For this review, take the finished solid that the model builds, in its own axes (mm). A direction names the side the tool comes from. Coordinates: 2 decimals unless noted, no trailing zeros. Loops run counter-clockwise (first coordinate to the right, second up) from the corner with the lowest first, then second, coordinate; pieces in that order, holes last.
1. Machinability: for faces 1 (the face through (-28.314, -11.099, -1.075)), 2 (the face through (37.676, 0.154, -22.737)), 3 (the face through (1, -1, -22)), which of the approach directions +Z, -Z, +X, -X, +Y, -Y give a long, thin tool a straight path to every point of the face, cutting with its end or side? Answer none if there is none.
2. Mouldability with a two-part tool opening along Z and no side actions: class faces 4 (the face through (23.38, 5.96, 8.44)), 5 (the face through (-31.66, 0.15, -22.96)), 6 (the face through (-0.27, -1.22, 18.77)) as pulls with the +Z half, pulls with the -Z half, needs draft (parallel to the pull), parting line crosses it, or undercut.
3. Take a section at B-B, the plane y = 0. Count the separate pieces of the cut face and the enclosed holes in it, then the cut area to 3 significant figures.
4. Clearance check with flat-ended pins moving along their axes: P1, Ø1.5, axis at y = 11, z = -7, coming from the -X side; P2, Ø6, axis at y = 4.5, z = 18.5, coming from the +X side; P3, Ø5.5, axis at x = 0, y = 0, coming from the -Z side. State where each tip first meets the part, or that it passes through.
5. To check wall thickness, follow probe 1 along Z at (x, y) = (0, 6); probe 2 along Z at (x, y) = (0, 1.75); probe 3 along X at (y, z) = (-12.7, 0). State the ranges of each line that lie inside material, in increasing order.
6. Take a section at A-A, the plane x = 0. State the section outline as (y, z) points.
```python
from build123d import *

# Parameters (mm, degrees)
SKETCH1_R               = 15.5
BOSS_EXTRUDE1_DEPTH     = 14
MOVE_START              = -14
MOVE_FACE1_DEPTH        = 28
CUT_EXTRUDE2_REACH      = 60.181
CUT_EXTRUDE2_END_RADIUS = 8.25
SKETCH5_R               = 2
SKETCH7_R               = 1.25
CUT_EXTRUDE3_DEPTH      = 68.268120394
FILLET1_R               = 8
CHAMFER1_SIZE           = 3
SKETCH8_R               = 3
CUT_EXTRUDE4_DEPTH      = 2


# Read off the part's stored shape, not the designer's step: Move Face1
with BuildPart() as part:
    # Sketch1 → Boss-Extrude1 (new, symmetric)
    with BuildSketch(Plane(origin=(0, 0, 0), x_dir=(1, 0, 0), z_dir=(0, 1, 0))):
        with BuildLine():
            Line((-32, 24), (32, 24))
            ThreePointArc((32, 24), (40, 0), (32, -24))
            Line((32, -24), (-32, -24))
            ThreePointArc((-32, -24), (-40, 0), (-32, 24))
        make_face()
        with Locations(Location((0, 0, 0), (0, 0, 270))):
            Circle(SKETCH1_R, mode=Mode.SUBTRACT)
    extrude(amount=BOSS_EXTRUDE1_DEPTH, both=True)

    # Sketch3 → Cut-Revolve1 (revolve, cut)
    with BuildSketch(Plane.XY):
        Polygon((-18, 2), (-19.432597466, 10.124663962), (-53.885297859, 4.049723325), (-52.452700394, -4.074940638), align=None)
    revolve(axis=Axis((-18, 2, 0), (-0.9848077530122092, -0.1736481776669237, 0)), mode=Mode.SUBTRACT)

    # Move Face1 outline → Move Face1 (add)
    with BuildSketch(Plane(origin=(0, 0, 0), x_dir=(1, 0, 0), z_dir=(0, 1, 0)).offset(MOVE_START)):
        with BuildLine():
            ThreePointArc((38.065732621, -24), (45, 0), (38.065732621, 24))
            Line((38.065732621, 24), (32, 24))
            ThreePointArc((32, 24), (40, 0), (32, -24))
            Line((32, -24), (38.065732621, -24))
        make_face()
    extrude(amount=MOVE_FACE1_DEPTH)

    # Sketch4 → Cut-Revolve2 (revolve, cut)
    with BuildSketch(Plane(origin=(0, 0, 0), x_dir=(0, -1, 0), z_dir=(-0.34202014332566943, 0, 0.9396926207859081)), mode=Mode.PRIVATE) as cut_revolve2_sk:
        Polygon((-6, 25), (-8.135257122, 32.968888067), (31.446035064, 43.574663343), (33.581292186, 35.605775277), align=None)
    cut_revolve2 = revolve(cut_revolve2_sk.sketch.rotate(Axis((23.49231552, 6, 8.550503583), (0.24321034680169487, -0.9659258262890681, 0.08852132690137743)), 160.629944791), axis=Axis((23.49231552, 6, 8.550503583), (0.24321034680169487, -0.9659258262890681, 0.08852132690137743)), mode=Mode.SUBTRACT)

    # Sketch6 → Cut-Revolve3 (revolve, cut)
    with BuildSketch(Plane(origin=(0, 0, 0), x_dir=(0, -1, 0), z_dir=(-0.34202014332566943, 0, 0.9396926207859081)), mode=Mode.PRIVATE) as cut_revolve3_sk:
        Polygon((4, 30), (6, 30), (6, 45), (6, 46), (2, 46), (2, 45), (2, 44), (4, 44), align=None)
    cut_revolve3 = revolve(cut_revolve3_sk.sketch.rotate(Axis((28.190778624, -6, 10.2606043), (0.9396926207859081, 0, 0.3420201433256695)), 90), axis=Axis((28.190778624, -6, 10.2606043), (0.9396926207859081, 0, 0.3420201433256695)), mode=Mode.SUBTRACT)

    # Mirror1: Cut-Revolve2, Cut-Revolve3 across plane
    add(cut_revolve2.mirror(Plane.XY), mode=Mode.SUBTRACT)
    add(cut_revolve3.mirror(Plane.XY), mode=Mode.SUBTRACT)

    # Cut-Extrude2: up to this cylinder (the profile starts outside it)
    cut_extrude2_end = Plane(origin=(-32.374316871, -0.534579894, 0), z_dir=(0.9848077530122092, 0.1736481776669237, 0)) * Cylinder(CUT_EXTRUDE2_END_RADIUS, 137.862, mode=Mode.PRIVATE)
    # Sketch5 → Cut-Extrude2 (cut, up to the surface)
    with BuildSketch(Plane.XZ.offset(14), mode=Mode.PRIVATE) as cut_extrude2_sk1:
        with Locations(Location((-30, 0, 0), (0, 0, 270))):
            Circle(SKETCH5_R)
    cut_extrude2_tool1 = extrude(cut_extrude2_sk1.sketch, amount=-CUT_EXTRUDE2_REACH, mode=Mode.PRIVATE) - cut_extrude2_end
    add(cut_extrude2_tool1.solids().sort_by_distance((-30, -14, 0))[0], mode=Mode.SUBTRACT)

    # Sketch7 → Cut-Extrude3 (cut, through all)
    with BuildSketch(Plane.XY.offset(24)):
        Circle(SKETCH7_R)
    extrude(amount=-CUT_EXTRUDE3_DEPTH, mode=Mode.SUBTRACT)

    # Fillet1
    fillet1_edges = [part.edges().sort_by_distance(p)[0] for p in [
        (-32, 0, -24),
        (38.065732621, 0, -24),
        (38.065732621, 0, 24),
        (-32, 0, 24),
    ]]
    fillet(fillet1_edges, radius=FILLET1_R)

    # Chamfer1
    chamfer1_edges = [part.edges().sort_by_distance(p)[0] for p in [
        (2.824420857, -14, -24),
        (2.824420857, 14, -24),
        (-40, -14, 0),
        (45, -14, 0),
        (2.824420857, -14, 24),
        (-31.712812921, -14, 22.92820323),
        (-31.712812921, -14, -22.92820323),
        (37.623363466, -14, 22.770364675),
        (37.623363466, -14, -22.770364675),
        (45, 14, 0),
        (-40, 14, 0),
        (2.824420857, 14, 24),
        (-31.712812921, 14, 22.92820323),
        (-31.712812921, 14, -22.92820323),
        (37.623363466, 14, 22.770364675),
        (37.623363466, 14, -22.770364675),
    ]]
    chamfer(chamfer1_edges, length=CHAMFER1_SIZE)

    # Sketch8 → Cut-Extrude4 (cut)
    with BuildSketch(Plane.XY.offset(24)):
        Circle(SKETCH8_R)
    cut_extrude4 = extrude(amount=-CUT_EXTRUDE4_DEPTH, mode=Mode.SUBTRACT)

    # Mirror2: Cut-Extrude4 across plane
    add(cut_extrude4.mirror(Plane.XY), mode=Mode.SUBTRACT)


solid = part.part
```
Results list:
1. face 1: -Y
1. face 2: -Z, +X, +Y, -Y
1. face 3: -Z
2. face 4: undercut
2. face 5: pulls with the -Z half
2. face 6: needs draft
3. separate pieces: 2
3. enclosed holes: 2
3. area: 2,220 mm2
4. P1: stops at x = -39.51
4. P2: stops at x = 42.25
4. P3: stops at z = -22
5. probe 1: z = -24 to -15.5, 15.5 to 24
5. probe 2: z = -22 to -15.5, 15.5 to 22
5. probe 3: x = -38.3 to -32, -28 to -15.5, 15.5 to 43.3
6. outline: (-14, -21) - (-11, -24) - (-3, -24) - (-3, -22) - (-1.25, -22) - (-1.25, -15.5) - (-14, -15.5) - close; (-14, 15.5) - (-1.25, 15.5) - (-1.25, 22) - (-3, 22) - (-3, 24) - (-11, 24) - (-14, 21) - close; (1.25, -22) - (3, -22) - (3, -24) - (11, -24) - (14, -21) - (14, -15.5) - (1.25, -15.5) - close; (1.25, 15.5) - (14, 15.5) - (14, 21) - (11, 24) - (3, 24) - (3, 22) - (1.25, 22) - close
